Source: CAD feature listing. Evaluate the final solid. Frame: model axes, mm. Face numbers are marked on the shaded views. A direction names the side the tool comes from. Round coordinates to 2 decimals unless told otherwise and drop trailing zeros. Order: outer loops, then holes, each group sorted by start corner. A loop starts at its lowest first (then second) coordinate and runs counter-clockwise, first axis right, second up. Notation, with made-up numbers: (-32.75, -38) -> (4.25, -38) arc R23 ccw to (4.25, 0) -> close; hole circle Ø3 at (-30.5, 47.25). An arc over 180 degrees is marked (long way). One line per item, written item: value. Start each with the question number.
1) Reachability of the marked faces 1, 2, 3 and 4 from +Z, -Z, +X, -X, +Y, -Y: full face, straight path, thin tool, end or side. Return the list, or none.
2) Section A-A (y = 239). Return the cut outline in (x, z).
3) Section B-B (x = 178.5). Return the cut outline in (y, z), and give its area (3 significant figures).
4) Section D-D (y = 53). Return the cut outline in (x, z).
5) Ray query, L1, parallel to X at y = 135, z = 150; L2, parallel to X at y = 135.75, z = 80; L3, parallel to X at y = 80.5, z = 109.5. Return the intervals inside material, ascending.
6) Section C-C (z = 80). Return the cut outline in (x, y).
7) Pin query (flat end, axial travel): P1, Ø20, axis at x = 75, z = 150, coming from the -Y side; P2, Ø1, axis at y = 169.5, z = 70.5, coming from the +X side; P3, Ø10, axis at x = 153.5, z = 148.5, coming from the +Y side; P4, Ø3, axis at y = -5, z = 103.5, coming from the -X side. Return the tip coordinate at first contact, or that it passes through.
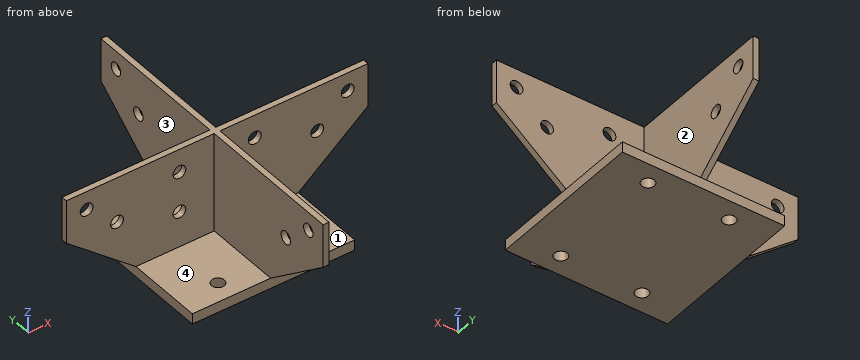
```python
from build123d import *

# Parameters (mm, degrees)
SKETCH_1_W                  = 280
SKETCH_1_H                  = 274
EXTRUDE_1_DEPTH             = 18
SKETCH_2_W                  = 520
SKETCH_2_H                  = 10
EXTRUDE_2_DEPTH             = 172
SKETCH_3_W                  = 10
SKETCH_3_H                  = 520
EXTRUDE_3_DEPTH             = 172
CUT_EXTRUDE_1_DEPTH         = 514.745072969
CUT_EXTRUDE_2_DEPTH         = 514.745072969
CUT_EXTRUDE_3_DEPTH         = 517.066856134
CUT_EXTRUDE_4_DEPTH         = 517.066856134
SKETCH_9_R                  = 11.000000001
SKETCH_9_R_2                = 11
CUT_EXTRUDE_5_DEPTH         = 517.066856134
SKETCH_10_R                 = 11
CUT_EXTRUDE_6_DEPTH         = 514.745072969
SKETCH_11_R                 = 11
CUT_EXTRUDE_7_DEPTH         = 595.734394499
PATTERN_LINEAR_1_COUNT      = 2
PATTERN_LINEAR_1_PITCH      = 140
PATTERN_LINEAR_1_COUNT_DIR2 = 2
PATTERN_LINEAR_1_PITCH_DIR2 = 204


with BuildPart() as part:
    # 草图1 → 拉伸1 (new body)
    with BuildSketch(Plane.XY):
        with Locations((140, 137)):
            Rectangle(SKETCH_1_W, SKETCH_1_H)
    extrude(amount=EXTRUDE_1_DEPTH)

    # 草图2 → 拉伸2 (add)
    with BuildSketch(Plane.XY.offset(18)):
        with Locations((140, 137)):
            Rectangle(SKETCH_2_W, SKETCH_2_H)
    extrude(amount=EXTRUDE_2_DEPTH)

    # 草图3 → 拉伸3 (add)
    with BuildSketch(Plane.XY.offset(18)):
        with Locations((140, 137)):
            Rectangle(SKETCH_3_W, SKETCH_3_H)
    extrude(amount=EXTRUDE_3_DEPTH)

    # 草图4 → 切除-拉伸1 (cut, through all)
    with BuildSketch(Plane(origin=(145, 0, 0), x_dir=(0, 0, -1), z_dir=(1, 0, 0))):
        Polygon((-115, 397), (-18, 274), (-18, 397), align=None)
    extrude(amount=-CUT_EXTRUDE_1_DEPTH, mode=Mode.SUBTRACT)

    # 草图5 → 切除-拉伸2 (cut, through all)
    with BuildSketch(Plane.ZY.offset(-135)):
        Polygon((115, -123), (18, 0), (18, -123), align=None)
    extrude(amount=-CUT_EXTRUDE_2_DEPTH, mode=Mode.SUBTRACT)

    # 草图6 → 切除-拉伸3 (cut, through all)
    with BuildSketch(Plane(origin=(0, 142, 0), x_dir=(1, 0, 0), z_dir=(0, 1, 0))):
        Polygon((280, -18), (400, -115), (400, -18), align=None)
    extrude(amount=-CUT_EXTRUDE_3_DEPTH, mode=Mode.SUBTRACT)

    # 草图8 → 切除-拉伸4 (cut, through all)
    with BuildSketch(Plane(origin=(0, 142, 0), x_dir=(1, 0, 0), z_dir=(0, 1, 0))):
        Polygon((0, -18), (-120, -115), (-120, -18), align=None)
    extrude(amount=-CUT_EXTRUDE_4_DEPTH, mode=Mode.SUBTRACT)

    # 草图9 → 切除-拉伸5 (cut, through all)
    with BuildSketch(Plane.XZ.offset(-132)):
        with Locations(Location((-85.189055636, 158.240447361, 0), (0, 0, 270))):
            Circle(SKETCH_9_R)
        with Locations(Location((75, 150, 0), (0, 0, 270))):
            Circle(SKETCH_9_R_2)
        with Locations(Location((-32.636595866, 112, 0), (0, 0, 270))):
            Circle(SKETCH_9_R_2)
        with Locations(Location((75, 80, 0), (0, 0, 270))):
            Circle(SKETCH_9_R_2)
        with Locations(Location((205, 150, 0), (0, 0, 270))):
            Circle(SKETCH_9_R_2)
        with Locations(Location((205, 80, 0), (0, 0, 270))):
            Circle(SKETCH_9_R_2)
        with Locations(Location((365.189055636, 158.240447361, 0), (0, 0, 270))):
            Circle(SKETCH_9_R)
        with Locations(Location((312.636595866, 112, 0), (0, 0, 270))):
            Circle(SKETCH_9_R_2)
    extrude(amount=-CUT_EXTRUDE_5_DEPTH, mode=Mode.SUBTRACT)

    # 草图10 → 切除-拉伸6 (cut, through all)
    with BuildSketch(Plane(origin=(145, 0, 0), x_dir=(0, 0, -1), z_dir=(1, 0, 0))):
        with Locations(Location((-158.241096139, 362.189055636, 0), (0, 0, 90))):
            Circle(SKETCH_10_R)
        with Locations(Location((-112, 309.636595866, 0), (0, 0, 90))):
            Circle(SKETCH_10_R)
        with Locations(Location((-112, -35.636595866, 0), (0, 0, 90))):
            Circle(SKETCH_10_R)
        with Locations(Location((-158.241096139, -88.189055636, 0), (0, 0, 90))):
            Circle(SKETCH_10_R)
    extrude(amount=-CUT_EXTRUDE_6_DEPTH, mode=Mode.SUBTRACT)

    # 草图11 → 切除-拉伸7 (cut, through all)
    with BuildSketch(Plane(origin=(0, 0, 0), x_dir=(-1, 0, 0), z_dir=(0, 0, -1))):
        with Locations((-210, 35)):
            Circle(SKETCH_11_R)
    cut_extrude_7 = extrude(amount=-CUT_EXTRUDE_7_DEPTH, mode=Mode.SUBTRACT)

    # 阵列(线性)1: Cut-Extrude 7 2 × 2
    with Locations(*[(-i * PATTERN_LINEAR_1_PITCH, j * PATTERN_LINEAR_1_PITCH_DIR2, 0) for i in range(PATTERN_LINEAR_1_COUNT) for j in range(PATTERN_LINEAR_1_COUNT_DIR2) if (i, j) != (0, 0)]):
        add(cut_extrude_7, mode=Mode.SUBTRACT)


solid = part.part
```
Findings:
1. face 1: +Z, +X, -Y
1. face 2: +Z, +X, +Y
1. face 3: +Z, -X, +Y
1. face 4: +Z, -X, -Y
2. outline: (0, 0) -> (59, 0) -> (59, 18) -> (0, 18) -> close; (81, 0) -> (199, 0) -> (199, 18) -> (145, 18) -> (145, 190) -> (135, 190) -> (135, 18) -> (81, 18) -> close; (221, 0) -> (280, 0) -> (280, 18) -> (221, 18) -> close
3. outline: (0, 0) -> (274, 0) -> (274, 18) -> (142, 18) -> (142, 190) -> (132, 190) -> (132, 18) -> (0, 18) -> close
3. area: 6,650 mm2
4. outline: (0, 0) -> (280, 0) -> (280, 18) -> (145, 18) -> (145, 190) -> (135, 190) -> (135, 18) -> (0, 18) -> close
5. L1: -120 to -92.48, -77.9 to 64, 86 to 194, 216 to 357.9, 372.48 to 400
5. L2: -76.7 to 64, 86 to 194, 216 to 356.7
5. L3: 135 to 145
6. outline: (-76.7, 132) -> (64, 132) -> (64, 142) -> (-76.7, 142) -> close; (86, 132) -> (135, 132) -> (135, -78.62) -> (145, -78.62) -> (145, 132) -> (194, 132) -> (194, 142) -> (145, 142) -> (145, 352.62) -> (135, 352.62) -> (135, 142) -> (86, 142) -> close; (216, 132) -> (356.7, 132) -> (356.7, 142) -> (216, 142) -> close
7. P1: through
7. P2: x = 145
7. P3: y = 142
7. P4: x = 135
